The model under review builds one solid part; all positions refer to its coordinate system, in mm. Face numbers are marked on the shaded views. A direction names the side the tool comes from. Round coordinates to 2 decimals unless told otherwise and drop trailing zeros. Write each loop counter-clockwise with the first axis right and the second up, starting at its lowest first coordinate (ties: lowest second). Pieces come first, ordered by that corner, then holes. Notation, with made-up numbers: (-16.5, 10.5) -> (-0.5, 10.5) arc R26 cw to (-0.5, 31.5) -> close; hole circle Ø6 at (52.25, 88). An arc over 180 degrees is marked (long way). Answer as a JSON object with one key per item and string values. Group by question number.
1) We need section D-D, the plane x = 8.5. Write out the cut boundary in (y, z).
2) We need section B-B, the plane z = -8. Write out the cut boundary in (x, y).
3) To check wall thickness, follow probe 1 along Z at (x, y) = (58, 23.25); probe 2 along Y at (x, z) = (62, 15); probe 3 along Y at (x, z) = (7, -67). State the ranges of each line that lie inside material, in increasing order. Write a range as [from, to].
4) We need section A-A, the plane x = 62. Write out the cut boundary in (y, z), then the cut area to 3 significant figures.
5) Insertion check: pin 1 Ø15 at (x, y) = (49, 7.5) entering from +Z; pin 2 Ø7.5 at (x, y) = (65, 17.5) entering from -Z. Each pin has a flat end and moves straight along its axis. Give the tip position at first contact, or say it passes through.
6) We need section C-C, the plane z = 51. Write out the cut boundary in (x, y), then the cut area to 3 significant figures.
7) Mouldability with a two-part tool opening along X and no side actions: class the marked faces 1, 2 and 3 as pulls with the +X half, pulls with the -X half, needs draft (parallel to the pull), parting line crosses it, or undercut.
8) Machinability: for the marked faces 4 and 5, which of the approach directions +Z, -Z, +X, -X, +Y, -Y give a long, thin tool a straight path to every point of the face, cutting with its end or side? Answer none if there is none.
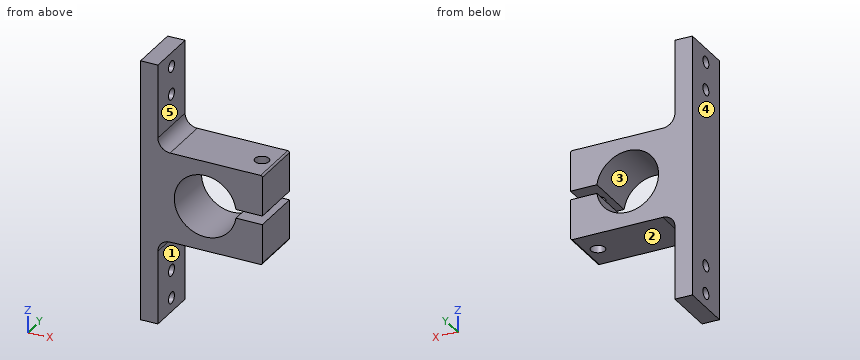
from build123d import *

# Parameters (mm, degrees)
SKETCH4_R                        = 17.8
BOSS_EXTRUDE2_DEPTH              = 30
SKETCH6_W                        = 21.036522063
SKETCH6_H                        = 5
CUT_EXTRUDE3_DEPTH               = 107.887791632
SKETCH7_R                        = 4
KIRISTYSRUUVI_M8_DEPTH           = 127.335426544
SKETCH9_R                        = 3.25
PROFIILN_KIINNITYSREI_T_M6_DEPTH = 101.623058987
FILLET1_R                        = 7
FILLET2_R                        = 1


with BuildPart() as part:
    # Sketch4 → Boss-Extrude2 (new body)
    with BuildSketch(Plane(origin=(0, 0, 0), x_dir=(1, 0, 0), z_dir=(0, 1, 0))):
        Polygon((0, 75), (10, 75), (10, 25.8), (70, 25.8), (70, -25.8), (10, -25.8), (10, -75), (0, -75), align=None)
        with Locations(Location((37.2, 0, 0), (0, 0, 270))):
            Circle(SKETCH4_R, mode=Mode.SUBTRACT)
    extrude(amount=BOSS_EXTRUDE2_DEPTH)

    # Sketch6 → Cut-Extrude3 (cut, through all)
    with BuildSketch(Plane(origin=(0, 30, 0), x_dir=(1, 0, 0), z_dir=(0, 1, 0))):
        with Locations((59.481738968, 0)):
            Rectangle(SKETCH6_W, SKETCH6_H)
    extrude(amount=-CUT_EXTRUDE3_DEPTH, mode=Mode.SUBTRACT)

    # Sketch7 → Kiristysruuvi M8 (cut, through all)
    with BuildSketch(Plane.XY.offset(25.8)):
        with Locations((62, 15)):
            Circle(SKETCH7_R)
    extrude(amount=-KIRISTYSRUUVI_M8_DEPTH, mode=Mode.SUBTRACT)

    # Sketch9 → Profiiln kiinnitysreiät M6 (cut, through all)
    with BuildSketch(Plane(origin=(10, 0, 0), x_dir=(0, 0, -1), z_dir=(1, 0, 0))):
        with Locations((-67, 15)):
            Circle(SKETCH9_R)
        with Locations((-51, 15)):
            Circle(SKETCH9_R)
        with Locations(Location((67, 15, 0), (0, 0, 180))):
            Circle(SKETCH9_R)
        with Locations(Location((51, 15, 0), (0, 0, 180))):
            Circle(SKETCH9_R)
    extrude(amount=-PROFIILN_KIINNITYSREI_T_M6_DEPTH, mode=Mode.SUBTRACT)

    # Fillet1
    fillet1_edges = [part.edges().sort_by_distance(p)[0] for p in [
        (10, 15, -25.8),
        (10, 15, 25.8),
    ]]
    fillet(fillet1_edges, radius=FILLET1_R)

    # Fillet2
    fillet2_edges = [part.edges().sort_by_distance(p)[0] for p in [
        (70, 15, -25.8),
        (70, 15, 25.8),
    ]]
    fillet(fillet2_edges, radius=FILLET2_R)


solid = part.part
Here are the results:
{
 "1": {"outline": "(0, -75) -> (30, -75) -> (30, 75) -> (0, 75) -> close; hole circle Ø6.5 at (15, -67); hole circle Ø6.5 at (15, -51); hole circle Ø6.5 at (15, 51); hole circle Ø6.5 at (15, 67)"},
 "2": {"outline": "(0, 0) -> (21.3, 0) -> (21.3, 30) -> (0, 30) -> close; (53.1, 0) -> (70, 0) -> (70, 30) -> (53.1, 30) -> close; hole circle Ø8 at (62, 15)"},
 "3": {"probe 1": "z = [-25.8, -2.5], [2.5, 25.8]", "probe 2": "y = [0, 11], [19, 30]", "probe 3": "y = [0, 11.75], [18.25, 30]"},
 "4": {"outline": "(0, -25.8) -> (11, -25.8) -> (11, -2.5) -> (0, -2.5) -> close; (0, 2.5) -> (11, 2.5) -> (11, 25.8) -> (0, 25.8) -> close; (19, -25.8) -> (30, -25.8) -> (30, -2.5) -> (19, -2.5) -> close; (19, 2.5) -> (30, 2.5) -> (30, 25.8) -> (19, 25.8) -> close", "area": "1,030 mm^2"},
 "5": {"pin 1": "stops at z = 25.8", "pin 2": "stops at z = -25.8"},
 "6": {"outline": "(0, 0) -> (10, 0) -> (10, 11.75) -> (0, 11.75) -> close; (0, 18.25) -> (10, 18.25) -> (10, 30) -> (0, 30) -> close", "area": "235 mm^2"},
 "7": {"face 1": "pulls with the +X half", "face 2": "needs draft", "face 3": "undercut"},
 "8": {"face 4": "+Z, -Z, -X, +Y, -Y", "face 5": "+Z, +X, +Y, -Y"}
}
